Job drawing, mm, ordinate dimensions from the low corner. One solid piece. Give positions to 0.01 mm unless a question says otherwise; leave off trailing zeros. Order: outer loops, then holes, each group sorted by start corner. A loop starts at its lowest first (then second) coordinate and runs counter-clockwise, first axis right, second up.
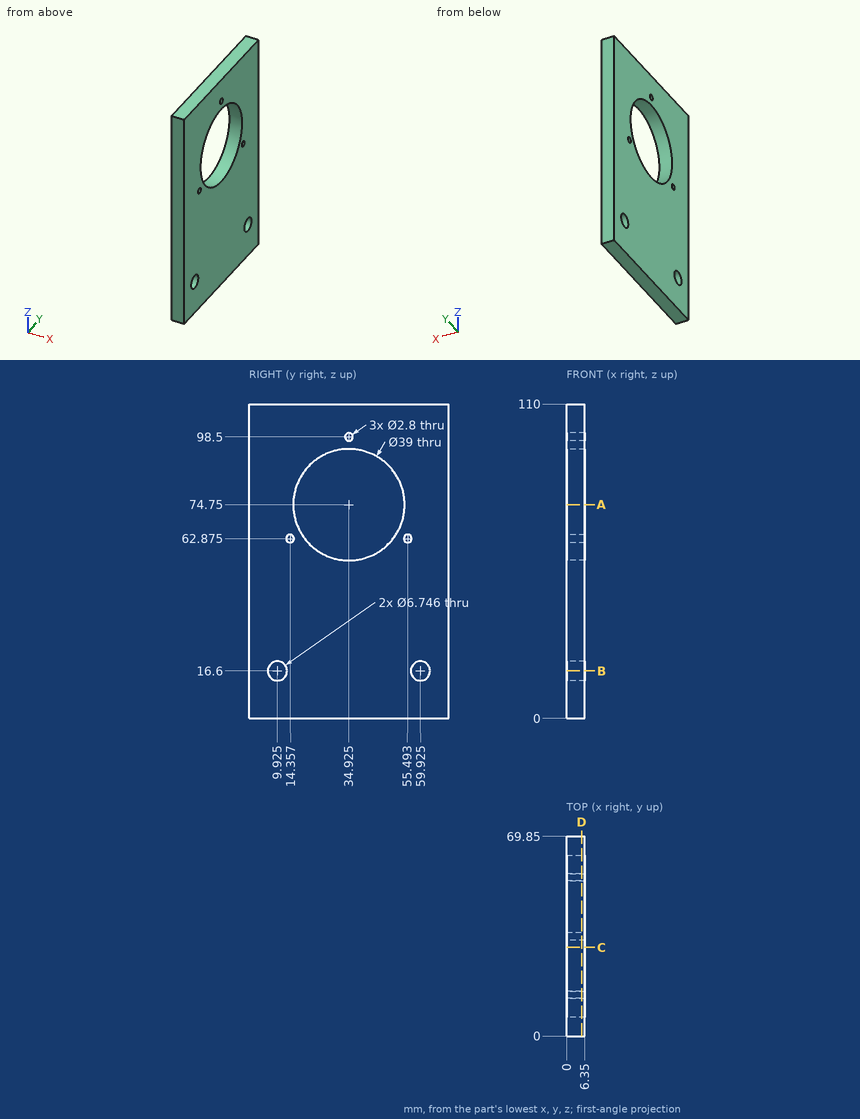
Item 1: Band-saw the part on C-C on y = 31. List the corners of the cut face in (x, z), plus the area to 3 significant figures.
Item 2: Drill centre lines: probe 1 along Z at (x, y) = (2.5, 9); probe 2 along Z at (x, y) = (3, 41); probe 3 along Y at (x, z) = (3.5, 99). Where is each one in solid material? Low to high.
Item 3: Band-saw the part on D-D on x = 5.25. Give the number of separate pieces and of enclosed holes in the cut face, plus the area to 3 significant figures.
Item 4: Band-saw the part on B-B on z = 16.6. List the corners of the cut face in (x, y).
Item 5: Band-saw the part on A-A on z = 74.75. List the corners of the cut face in (x, y) (3 decimals), plus the area to 3 significant figures.
Working result:
1. outline: (0, 0) - (6.35, 0) - (6.35, 55.65) - (0, 55.65) - close; (0, 93.85) - (6.35, 93.85) - (6.35, 110) - (0, 110) - close
1. area: 456 mm2
2. probe 1: z = 0 to 13.36, 19.84 to 110
2. probe 2: z = 0 to 56.22, 93.28 to 110
2. probe 3: y = 0 to 33.62, 36.23 to 69.85
3. separate pieces: 1
3. enclosed holes: 6
3. area: 6,400 mm2
4. outline: (0, 0) - (6.35, 0) - (6.35, 6.55) - (0, 6.55) - close; (0, 13.3) - (6.35, 13.3) - (6.35, 56.55) - (0, 56.55) - close; (0, 63.3) - (6.35, 63.3) - (6.35, 69.85) - (0, 69.85) - close
5. outline: (0, 0) - (6.35, 0) - (6.35, 15.425) - (0, 15.425) - close; (0, 54.425) - (6.35, 54.425) - (6.35, 69.85) - (0, 69.85) - close
5. area: 196 mm2
